The model under review builds one solid part; all positions refer to its coordinate system, in mm. Face numbers are marked on the shaded views. Coordinates: 2 decimals unless noted, no trailing zeros. Order: outer loops, then holes, each group sorted by start corner. A loop starts at its lowest first (then second) coordinate and runs counter-clockwise, first axis right, second up. Notation, with made-up numbers: M 20,-29.75 L 59,-29.75 A16 cw 59,-20.75 Z; hole C -12.75,-10 d4. An arc over 180 degrees is marked long. One line per item, written item: value.
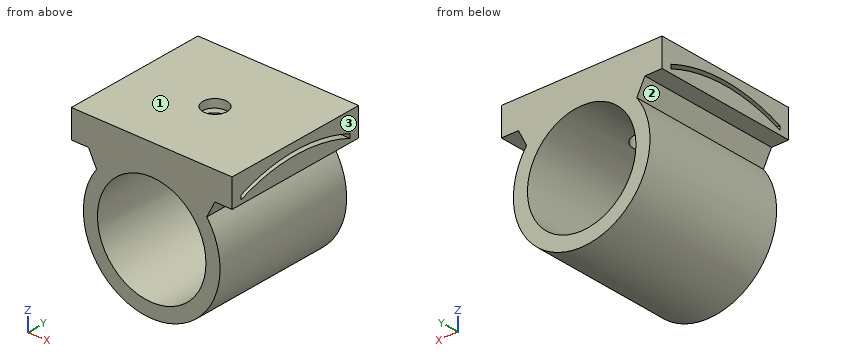
```python
from build123d import *

# Parameters (mm, degrees)
F0_R         = 8.5
F1_DEPTH     = 18
F2_R         = 6.75
F3_DEPTH     = 18
F4_W         = 18
F4_H         = 3.5
F5_DEPTH     = 10
F7_DEPTH     = 20
F8_R         = 1.5
F9_DEPTH     = 5
F10_T1_DEPTH = 18


# Not quite as in the source:
# - a fillet or chamfer that OpenCascade refuses, or shapes differently, is made with other operations: its cross-section is extruded or revolved along the edge and cut away or added


with BuildPart() as f1:
    # F0 (on Front) → F1 (new body)
    with BuildSketch(Plane.XZ):
        Circle(F0_R)
    extrude(amount=F1_DEPTH)

    # F2 (on face) → F3 (cut, through all)
    with BuildSketch(Plane.XZ.offset(18)):
        Circle(F2_R)
    extrude(amount=-F3_DEPTH, mode=Mode.SUBTRACT)

    # F4 (on Right) → F5 (join, symmetric)
    with BuildSketch(Plane.YZ):
        with Locations((-9, 8.75)):
            Rectangle(F4_W, F4_H)
    extrude(amount=F5_DEPTH, both=True)

    # F6 (on face) → F7 (cut, through all)
    with BuildSketch(Plane.YZ.offset(10)):
        with BuildLine():
            Line((-16.75, 8), (-16.75, 7.5))
            ThreePointArc((-16.75, 7.5), (-9, 9), (-1.25, 7.5))
            Line((-1.25, 7.5), (-1.25, 8))
            ThreePointArc((-1.25, 8), (-9, 9.5), (-16.75, 8))
        make_face()
    extrude(amount=-F7_DEPTH, mode=Mode.SUBTRACT)

    # F8 (on face) → F9 (cut)
    with BuildSketch(Plane.XY.offset(10.5)):
        with Locations((0, -9)):
            Circle(F8_R)
    extrude(amount=-F9_DEPTH, mode=Mode.SUBTRACT)

    # F10: chamfer of 4 on 2 edges, made by hand

    # F10_s2 → F10_t1 (join)
    with BuildSketch(Plane.XZ):
        with BuildLine():
            Line((-6.7863990228, 4.8779762725), (-7.9352464288, 7.1426903404))
            Line((-7.9352464288, 7.1426903404), (-7.9352464288, 7.2226903404))
            ThreePointArc((-7.9352464288, 7.2226903404), (-6.3785359046, 7.08), (-4.8218253805, 7.08))
            Line((-4.8218253805, 7.08), (-4.7764434946, 6.9341176471))
            ThreePointArc((-4.7764434946, 6.9341176471), (-5.8850678371, 6.0218250184), (-6.7218457694, 4.8307229397))
            Line((-6.7218457694, 4.8307229397), (-6.7863990228, 4.8779762725))
        make_face()
        with BuildLine():
            Line((6.7863990228, 4.8779762725), (7.9352464288, 7.1426903404))
            Line((7.9352464288, 7.1426903404), (7.9352464288, 7.2226903404))
            ThreePointArc((7.9352464288, 7.2226903404), (6.3785359046, 7.08), (4.8218253805, 7.08))
            Line((4.8218253805, 7.08), (4.7764434946, 6.9341176471))
            ThreePointArc((4.7764434946, 6.9341176471), (5.8850678371, 6.0218250184), (6.7218457694, 4.8307229397))
            Line((6.7218457694, 4.8307229397), (6.7863990228, 4.8779762725))
        make_face()
    extrude(amount=F10_T1_DEPTH)


solid = f1.part
```
(1) We need section B-B, the plane x = -3.75. State the section outline as (y, z) points.
Geometry results:
outline: M -18,-7.63 L 0,-7.63 L 0,-5.61 L -18,-5.61 Z; M -18,5.61 L 0,5.61 L 0,10.5 L -18,10.5 Z; hole M -16.75,7.5 A20.77 cw -1.25,7.5 L -1.25,8 A20.77 ccw -16.75,8 Z
(2) For L1, parallel to Z at x = 4, y = -2; L2, parallel to Y at x = 0, z = 9.95; L3, parallel to X at y = -9, z = 8.25, list the stretches that pass through material, from the lowest coordinate up.
Geometry results:
L1: z = -7.5 to -5.44, 5.44 to 7.78, 8.28 to 10.5
L2: y = -18 to -10.5, -7.5 to 0
L3: x = -10 to -1.5, 1.5 to 10
(3) Insertion check: pin 1 Ø0.6 at (x, y) = (9, -5.5) entering from -Z; pin 2 Ø2 at (x, y) = (2, -7) entering from -Z; pin 3 Ø1.5 at (x, y) = (4, -11.5) entering from -Z. Each pin has a flat end and moves straight along its axis. Give the tip position at first contact, or say it passes through.
Geometry results:
pin 1: stops at z = 7
pin 2: stops at z = -8.44
pin 3: stops at z = -7.85
(4) Mouldability with a two-part tool opening along Z and no side actions: class the marked faces 1, 2 and 3 as +Z half, -Z half, draft (parallel to the pull), parting line (faces both ways), or undercut.
Geometry results:
face 1: +Z half
face 2: undercut
face 3: draft
(5) We need section A-A, the plane y = -9. State the section outline as (x, z) points.
Geometry results:
outline: M -10,7 L -7.86,7 L -6.86,5.02 A8.5 ccw long 6.86,5.02 L 7.86,7 L 10,7 L 10,9 L 1.5,9 L 1.5,6.58 A6.75 cw long -1.5,6.58 L -1.5,9 L -10,9 Z; M -10,9.5 L -1.5,9.5 L -1.5,10.5 L -10,10.5 Z; M 1.5,9.5 L 10,9.5 L 10,10.5 L 1.5,10.5 Z
(6) We need section D-D, the plane z = -3. State the section outline as (x, y) points.
Geometry results:
outline: M -7.95,-18 L -6.05,-18 L -6.05,0 L -7.95,0 Z; M 6.05,-18 L 7.95,-18 L 7.95,0 L 6.05,0 Z
(7) We need section C-C, the plane y = -2.5. State the section outline as (x, z) points, plus the area to 3 significant figures.
Geometry results:
outline: M -10,7 L -7.86,7 L -6.86,5.02 A8.5 ccw long 6.86,5.02 L 7.86,7 L 10,7 L 10,7.96 L -10,7.96 Z; M -10,8.46 L 10,8.46 L 10,10.5 L -10,10.5 Z; hole C 0,0 d13.5
area: 140 mm2
